```python
from build123d import *

# Parameters (mm, degrees)
EXTRUDE_THIN2_DEPTH = 15
SKETCH6_R           = 4.25
CUT_EXTRUDE1_DEPTH  = 55.927224579
FILLET1_R           = 10


with BuildPart() as part:
    # Sketch1 → Extrude-Thin2 (new body)
    with BuildSketch(Plane.XY):
        with BuildLine():
            Line((46, 0), (26, 0))
            ThreePointArc((26, 0), (0, 26), (-26, 0))
            Line((-26, 0), (-46, 0))
            Line((-46, 0), (-46, 2))
            Line((-46, 2), (-27.928480088, 2))
            ThreePointArc((-27.928480088, 2), (0, 28), (27.928480088, 2))
            Line((27.928480088, 2), (46, 2))
            Line((46, 2), (46, 0))
        make_face()
    extrude(amount=-EXTRUDE_THIN2_DEPTH)

    # Sketch6 → Cut-Extrude1 (cut, through all)
    with BuildSketch(Plane(origin=(0, 2, 0), x_dir=(1, 0, 0), z_dir=(0, 1, 0))):
        with Locations(Location((-34.25, 7.5, 0), (0, 0, 180))):
            Circle(SKETCH6_R)
        with Locations(Location((34.25, 7.5, 0), (0, 0, 180))):
            Circle(SKETCH6_R)
    extrude(amount=-CUT_EXTRUDE1_DEPTH, mode=Mode.SUBTRACT)

    # Fillet1
    # the kernel refuses this fillet: 10 mm, written as the material it takes off along each edge
    with BuildSketch(Plane(origin=(-46, -25, -15), x_dir=(1, 0, 0), z_dir=(0, 1, 0)), Plane(origin=(46, 27, -15), x_dir=(-1, 0, 0), z_dir=(0, -1, 0))) as fillet1_piece_1:
        with BuildLine():
            CenterArc((FILLET1_R, -FILLET1_R), FILLET1_R, 90, 90)
            Line((0, -FILLET1_R), (0, 0))
            Line((0, 0), (FILLET1_R, 0))
        make_face()
    extrude(amount=52, mode=Mode.SUBTRACT)
    with BuildSketch(Plane(origin=(-46, -25, 0), x_dir=(1, 0, 0), z_dir=(0, 1, 0)), Plane(origin=(46, 27, 0), x_dir=(-1, 0, 0), z_dir=(0, -1, 0))) as fillet1_piece_2:
        with BuildLine():
            CenterArc((FILLET1_R, FILLET1_R), FILLET1_R, 180, 90)
            Line((0, FILLET1_R), (0, 0))
            Line((0, 0), (FILLET1_R, 0))
        make_face()
    extrude(amount=52, mode=Mode.SUBTRACT)


solid = part.part
```
The listing builds one solid part. Answer for the finished solid, in the listing's coordinates (mm). A direction names the side the tool comes from. Give positions to 0.01 mm unless a question says otherwise; leave off trailing zeros. Order: outer loops, then holes, each group sorted by start corner. A loop starts at its lowest first (then second) coordinate and runs counter-clockwise, first axis right, second up. Notation, with made-up numbers: (-4.5, -20) -> (53.5, -20) arc R31 ccw to (53.5, 18) -> close; hole circle Ø5 at (34, 10.5). An arc over 180 degrees is marked (long way). One line per item, written item: value.
1) Find section A-A, the plane x = 34.25. Determine the outline of the cut face in (y, z), plus the area to 3 significant figures.
Reported:
outline: (0, -15) -> (2, -15) -> (2, -11.75) -> (0, -11.75) -> close; (0, -3.25) -> (2, -3.25) -> (2, 0) -> (0, 0) -> close
area: 13.0 mm^2
2) Find section B-B, the plane y = 8.75. Determine the outline of the cut face in (x, z), plus the area to 3 significant figures.
Reported:
outline: (-26.6, -15) -> (-24.48, -15) -> (-24.48, 0) -> (-26.6, 0) -> close; (24.48, -15) -> (26.6, -15) -> (26.6, 0) -> (24.48, 0) -> close
area: 63.4 mm^2
3) Flat-ended cylindrical pins translate along their axes: P1, Ø2, axis at x = -13, y = 25, coming from the +Z side; P2, Ø4.5, axis at x = -35.5, z = -9.5, coming from the +Y side; P3, Ø1, axis at y = 13, z = -12, coming from the +X side; P4, Ø5, axis at x = -26.5, z = -12, coming from the +Y side. Find the tip coordinate at first contact, or state that the pin passes through.
Reported:
P1: stops at z = 0
P2: stops at y = 2
P3: stops at x = 25.05
P4: stops at y = 14.42
4) A tool of negligible diameter and unlimited length cuts with its end or side. For faces 1 (the flat face through (-38, 0, -11)), 2 (the flat face through (-39, 2, -7)), 3 (the flat face through (39, 2, -7)), from which of +Z, -Z, +X, -X, +Y, -Y can it reach the whole face along a straight path? Write none if from no direction.
Reported:
face 1: +Z, -Z, +X, -X, -Y
face 2: +Z, -Z, -X, +Y
face 3: +Z, -Z, +X, +Y
5) Find section D-D, the plane x = 7.5. Determine the outline of the cut face in (y, z).
Reported:
outline: (24.89, -15) -> (26.98, -15) -> (26.98, 0) -> (24.89, 0) -> close
6) Find the intervals of material crossed by line 1 (Z direction, x = -34.25, y = 1.15); line 2 (X direction, y = 13.5, z = -12.25); line 3 (Y direction, x = 28, z = -8.75), in increasing order.
Reported:
line 1: z = -15 to -11.75, -3.25 to 0
line 2: x = -24.53 to -22.22, 22.22 to 24.53
line 3: y = 0 to 2
7) Determine the mould class of faces 4 (the cylindrical face through (-30.88, 1.01, -10.09)), 5 (the cylindrical face through (-0.588, 27.994, -7.395)), 6 (the cylindrical face through (42, 1, -13)) for opening direction X: pulls with the +X half, pulls with the -X half, needs draft (parallel to the pull), parting line crosses it, or undercut.
Reported:
face 4: undercut
face 5: parting line crosses it
face 6: pulls with the +X half
8) Find section C-C, the plane z = -1.25. Determine the outline of the cut face in (x, y), plus the area to 3 significant figures.
Reported:
outline: (-40.84, 0) -> (-26, 0) arc R26 cw to (26, 0) -> (40.84, 0) -> (40.84, 2) -> (27.93, 2) arc R28 ccw to (-27.93, 2) -> (-40.84, 2) -> close
area: 221 mm^2
